Input: part model. Units: mm. Frame: model coordinates. A direction names the side the tool comes from. Give positions to 0.01 mm unless a question says otherwise; leave off trailing zeros. Order: outer loops, then holes, each group sorted by start corner. A loop starts at its lowest first (then second) coordinate and runs counter-clockwise, first axis right, second up. Notation, with made-up numbers: (70.25, 64.5) - (102.25, 64.5) arc R22 cw to (102.25, 88.5) - close; hole circle Ø9 at (5, 80.25). An arc over 180 degrees is marked (long way). Use a Markdown table: item, result.
from build123d import *

# Parameters (mm, degrees)
PARED_B_CHUMACERA_J2_START          = -21.35
CROQUIS1_W                          = 76
CROQUIS1_H                          = 81.25
PARED_B_CHUMACERA_J2_DEPTH          = 6.35
PARED_B_CHUMACERA_J2_REDONDEO_START = -21.35
CROQUIS2_R                          = 38
PARED_B_CHUMACERA_J2_REDONDEO_DEPTH = 6.35
PASO_PIN_Y_ROSCA_M4_EJEFALSO_START  = -21.35
CROQUIS3_R                          = 3.5
CROQUIS3_R_2                        = 1.65
PASO_PIN_Y_ROSCA_M4_EJEFALSO_DEPTH  = 6.35
ROSCA_M3_ESCUADRAS_START            = -21.35
CROQUIS4_R                          = 1.25
ROSCA_M3_ESCUADRAS_DEPTH            = 6.35
PASADORES_D4_START                  = 90.2
CROQUIS5_R                          = 2
PASADORES_D4_DEPTH                  = 8
ROSCA_M3_BASES_CINCHO_START         = -21.35
CROQUIS6_R                          = 1.25
ROSCA_M3_BASES_CINCHO_DEPTH         = 6.35
PASO_M3_ESCUADRAS_TUERCA_START      = -21.35
CROQUIS7_R                          = 1.7
PASO_M3_ESCUADRAS_TUERCA_DEPTH      = 6.35
PASO_M3_BASE_CINCHO_TUERCA_START    = -21.35
CROQUIS8_R                          = 1.7
PASO_M3_BASE_CINCHO_TUERCA_DEPTH    = 6.35


with BuildPart() as part:
    # Croquis1 → Pared_B_chumacera_J2 (new body)
    with BuildSketch(Plane(origin=(0, 0, 0), x_dir=(1, 0, 0), z_dir=(0, 1, 0)).offset(PARED_B_CHUMACERA_J2_START)):
        with Locations((0, -130.825)):
            Rectangle(CROQUIS1_W, CROQUIS1_H)
    extrude(amount=PARED_B_CHUMACERA_J2_DEPTH)

    # Croquis2 → Pared_B_chumacera_J2_redondeo (add)
    with BuildSketch(Plane(origin=(0, 0, 0), x_dir=(1, 0, 0), z_dir=(0, 1, 0)).offset(PARED_B_CHUMACERA_J2_REDONDEO_START)):
        with Locations((0, -171.45)):
            Circle(CROQUIS2_R)
    extrude(amount=PARED_B_CHUMACERA_J2_REDONDEO_DEPTH)

    # Croquis3 → Paso_pin_y_rosca_M4_ejefalso (cut)
    with BuildSketch(Plane(origin=(0, 0, 0), x_dir=(1, 0, 0), z_dir=(0, 1, 0)).offset(PASO_PIN_Y_ROSCA_M4_EJEFALSO_START)):
        with Locations(Location((0, -171.45, 0), (0, 0, 270))):
            Circle(CROQUIS3_R)
        with Locations(Location((0, -190.95, 0), (0, 0, 270))):
            Circle(CROQUIS3_R_2)
        with Locations(Location((0, -151.95, 0), (0, 0, 270))):
            Circle(CROQUIS3_R_2)
    extrude(amount=PASO_PIN_Y_ROSCA_M4_EJEFALSO_DEPTH, mode=Mode.SUBTRACT)

    # Croquis4 → Rosca_M3_escuadras (cut)
    with BuildSketch(Plane(origin=(0, 0, 0), x_dir=(1, 0, 0), z_dir=(0, 1, 0)).offset(ROSCA_M3_ESCUADRAS_START)):
        with Locations(Location((-25, -105.2, 0), (0, 0, 270))):
            Circle(CROQUIS4_R)
        with Locations(Location((25, -105.2, 0), (0, 0, 270))):
            Circle(CROQUIS4_R)
    extrude(amount=ROSCA_M3_ESCUADRAS_DEPTH, mode=Mode.SUBTRACT)

    # Croquis5 → Pasadores_D4 (cut)
    with BuildSketch(Plane.XY.offset(PASADORES_D4_START)):
        with Locations((-30, -18.175)):
            Circle(CROQUIS5_R)
        with Locations((30, -18.175)):
            Circle(CROQUIS5_R)
    extrude(amount=PASADORES_D4_DEPTH, mode=Mode.SUBTRACT)

    # Croquis6 → Rosca_M3_bases_cincho (cut)
    with BuildSketch(Plane(origin=(0, 0, 0), x_dir=(1, 0, 0), z_dir=(0, 1, 0)).offset(ROSCA_M3_BASES_CINCHO_START)):
        with Locations(Location((0, -117, 0), (0, 0, 270))):
            Circle(CROQUIS6_R)
    extrude(amount=ROSCA_M3_BASES_CINCHO_DEPTH, mode=Mode.SUBTRACT)

    # Croquis7 → Paso_M3_escuadras_tuerca (cut)
    with BuildSketch(Plane(origin=(0, 0, 0), x_dir=(1, 0, 0), z_dir=(0, 1, 0)).offset(PASO_M3_ESCUADRAS_TUERCA_START)):
        with Locations(Location((-25, -105.2, 0), (0, 0, 270))):
            Circle(CROQUIS7_R)
        with Locations(Location((25, -105.2, 0), (0, 0, 270))):
            Circle(CROQUIS7_R)
    extrude(amount=PASO_M3_ESCUADRAS_TUERCA_DEPTH, mode=Mode.SUBTRACT)

    # Croquis8 → Paso_M3_base_cincho_tuerca (cut)
    with BuildSketch(Plane(origin=(0, 0, 0), x_dir=(1, 0, 0), z_dir=(0, 1, 0)).offset(PASO_M3_BASE_CINCHO_TUERCA_START)):
        with Locations(Location((0, -117, 0), (0, 0, 270))):
            Circle(CROQUIS8_R)
    extrude(amount=PASO_M3_BASE_CINCHO_TUERCA_DEPTH, mode=Mode.SUBTRACT)


solid = part.part
1. Material intervals for line 1 along X through (y, z) = (-18.25, 105.2); line 2 along Y through (x, z) = (-30, 95.75) (3 decimals); line 3 along X through (y, z) = (-17, 171.45), sorted ascending.
Response:
| item | result |
|---|---|
| line 1 | x = -38 to -26.7, -23.3 to 23.3, 26.7 to 38 |
| line 2 | y = -21.35 to -20.175, -16.175 to -15 |
| line 3 | x = -38 to -3.5, 3.5 to 38 |
2. Section query D-D (z = 199.5). Return loops of the section in (x, y), then the cut area to 3 significant figures.
Response:
| item | result |
|---|---|
| outline | (-25.64, -21.35) - (25.64, -21.35) - (25.64, -15) - (-25.64, -15) - close |
| area | 326 mm^2 |
3. Pin query (flat end, axial travel): pin 1 (4.5 mm diameter, centred on x = -25, z = 105.2, fed in from +Y); pin 2 (2.5 mm diameter, centred on x = -30, y = -18.175, fed in from +Z); pin 3 (1 mm diameter, centred on x = -29, y = -19, fed in from +Z); pin 4 (2 mm diameter, centred on x = 30.5, y = -17.5, fed in from -Z). Return the tip coordinate at first contact, or that it passes through.
Response:
| item | result |
|---|---|
| pin 1 | stops at y = -15 |
| pin 2 | stops at z = 196.3 |
| pin 3 | stops at z = 196.58 |
| pin 4 | stops at z = 98.2 |
4. Mould query, pull axis X, two halves, no side actions, for faces 3 (the face through (-38, -18, 131)), 4 (the face through (-0.84, -18.22, 209.44)), 5 (the face through (-1, -21.35, 149)), 6 (the face through (0.07, -18.22, 150.3)). Classes: pulls with the +X half, pulls with the -X half, needs draft (parallel to the pull), parting line crosses it, or undercut.
Response:
| item | result |
|---|---|
| face 3 | pulls with the -X half |
| face 4 | parting line crosses it |
| face 5 | needs draft |
| face 6 | undercut |
5. Section query C-C (z = 151.95). Return loops of the section in (x, y), then the cut area to 3 significant figures.
Response:
| item | result |
|---|---|
| outline | (-38, -21.35) - (-1.65, -21.35) - (-1.65, -15) - (-38, -15) - close; (1.65, -21.35) - (38, -21.35) - (38, -15) - (1.65, -15) - close |
| area | 462 mm^2 |
6. Section query B-B (x = 0). Return loops of the section in (y, z).
Response:
| item | result |
|---|---|
| outline | (-21.35, 90.2) - (-15, 90.2) - (-15, 115.3) - (-21.35, 115.3) - close; (-21.35, 118.7) - (-15, 118.7) - (-15, 150.3) - (-21.35, 150.3) - close; (-21.35, 153.6) - (-15, 153.6) - (-15, 167.95) - (-21.35, 167.95) - close; (-21.35, 174.95) - (-15, 174.95) - (-15, 189.3) - (-21.35, 189.3) - close; (-21.35, 192.6) - (-15, 192.6) - (-15, 209.45) - (-21.35, 209.45) - close |
7. Set-up query: faces 1 (the face through (25.51, -18.22, 106.82)), 2 (the face through (30, -18, 98.2)). Return all of +Z, -Z, +X, -X, +Y, -Y with unobstructed straight access to the full face (end or side cutting, diameter ignored); none if empty.
Response:
| item | result |
|---|---|
| face 1 | +Y, -Y |
| face 2 | -Z |
8. Section query A-A (z = 117). Return loops of the section in (x, y), then the cut area to 3 significant figures.
Response:
| item | result |
|---|---|
| outline | (-38, -21.35) - (-1.7, -21.35) - (-1.7, -15) - (-38, -15) - close; (1.7, -21.35) - (38, -21.35) - (38, -15) - (1.7, -15) - close |
| area | 461 mm^2 |
